Work out the finished part from the listing and answer in its coordinate system (mm). A direction names the side the tool comes from. Round coordinates to 2 decimals unless told otherwise and drop trailing zeros. Write each loop counter-clockwise with the first axis right and the second up, starting at its lowest first coordinate (ties: lowest second). Pieces come first, ordered by that corner, then holes. Notation, with made-up numbers: (19.25, -2.5) -> (34.25, -2.5) arc R7 cw to (34.25, 2.5) -> close; hole circle Ø1 at (55, -15.5). An arc over 180 degrees is marked (long way). One line per question, with ' | ' between items. Start each with the question number.
```python
from build123d import *

# Parameters (mm, degrees)
SKETCH2_R           = 23
CUT_EXTRUDE1_DEPTH  = 5
CUT_EXTRUDE2_START  = -2
SKETCH3_R           = 23
CUT_EXTRUDE2_DEPTH  = 2
SKETCH4_R           = 6
BOSS_EXTRUDE2_DEPTH = 5
CUT_EXTRUDE3_DEPTH  = 5
SKETCH6_R           = 1.5
CUT_EXTRUDE4_DEPTH  = 3
SKETCH7_RX          = 4
SKETCH7_RY          = 2.5
CUT_EXTRUDE5_DEPTH  = 3
CIRPATTERN1_COUNT   = 12


with BuildPart() as part:
    # Sketch1 → Revolve1 (revolve)
    with BuildSketch(Plane(origin=(0, 0, 0), x_dir=(1, 0, 0), z_dir=(0, 1, 0)), mode=Mode.PRIVATE) as revolve1_sk:
        Polygon((-5, 25), (0.5, 25), (0.5, 26.5), (0, 26.5), (0, 28), (3, 28), (3, 26.5), (2.5, 26.5), (2.5, 25), (5, 25), (5, 0), (-5, 0), align=None)
    revolve(revolve1_sk.sketch.rotate(Axis((0, 0, 0), (1, 0, 0)), 180), axis=Axis((0, 0, 0), (1, 0, 0)))

    # Sketch2 → Cut-Extrude1 (cut)
    with BuildSketch(Plane(origin=(5, 0, 0), x_dir=(0, 0, -1), z_dir=(1, 0, 0))):
        Circle(SKETCH2_R)
    extrude(amount=-CUT_EXTRUDE1_DEPTH, mode=Mode.SUBTRACT)

    # Sketch3 → Cut-Extrude2 (cut)
    with BuildSketch(Plane.ZY.offset(5).offset(CUT_EXTRUDE2_START)):
        with Locations(Location((0, 0, 0), (0, 0, 180))):
            Circle(SKETCH3_R)
    extrude(amount=CUT_EXTRUDE2_DEPTH, mode=Mode.SUBTRACT)

    # Sketch4 → Boss-Extrude2 (add)
    with BuildSketch(Plane(origin=(0, 0, 0), x_dir=(0, 0, -1), z_dir=(1, 0, 0))):
        with Locations(Location((0, 0, 0), (0, 0, 180))):
            Circle(SKETCH4_R)
    extrude(amount=BOSS_EXTRUDE2_DEPTH)

    # Sketch5 → Cut-Extrude3 (cut)
    with BuildSketch(Plane(origin=(5, 0, 0), x_dir=(0, 0, -1), z_dir=(1, 0, 0))):
        with BuildLine():
            Line((-1.936491673, 3.5), (1.936491673, 3.5))
            ThreePointArc((1.936491673, 3.5), (0, -4), (-1.936491673, 3.5))
        make_face()
    extrude(amount=-CUT_EXTRUDE3_DEPTH, mode=Mode.SUBTRACT)

    # Sketch6 → Cut-Extrude4 (cut)
    with BuildSketch(Plane.ZY.offset(3)):
        Circle(SKETCH6_R)
    extrude(amount=-CUT_EXTRUDE4_DEPTH, mode=Mode.SUBTRACT)

    # Sketch7 → Cut-Extrude5 (cut)
    with BuildSketch(Plane(origin=(0, 0, 0), x_dir=(0, 0, -1), z_dir=(1, 0, 0))):
        with Locations(Location((0, 15), (0, 0, -90))):
            Ellipse(SKETCH7_RX, SKETCH7_RY)
    cut_extrude5 = extrude(amount=-CUT_EXTRUDE5_DEPTH, mode=Mode.SUBTRACT)

    # CirPattern1: Cut-Extrude5 ×12 about axis
    cirpattern1_axis = Axis((4.242640687, 0, 0), (-1, 0, 0))
    for i in range(1, CIRPATTERN1_COUNT):
        add(cut_extrude5.rotate(cirpattern1_axis, i * 360 / CIRPATTERN1_COUNT), mode=Mode.SUBTRACT)


solid = part.part
```
(1) A cutting plane is placed at D-D, the plane y = 0. Count the separate pieces of the cut face and the enclosed holes in it, then the cut area to 3 significant figures.
(2) A cutting plane is placed at C-C, the plane z = -21.5. Determine the outline of the cut face in (x, y).
(3) Consider L1, parallel to Y at x = -1.8, z = 0; L2, parallel to Z at x = -1.5, y = 14.5; L3, parallel to Z at x = -1.5, y = -9. Determine where each line is inside the solid, lowest interval first.
(4) Given pin 1 Ø16 at (y, z) = (2.5, 9.5) entering from -X; pin 2 Ø4 at (x, z) = (1.5, 7.5) entering from +Y; pin 3 Ø12 at (y, z) = (4.5, 20.5) entering from -X; pin 4 Ø6 at (x, y) = (1.5, -21.5) entering from -Z, each flat-ended and moving along its own axis, determine where each tip first touches the part or whether it passes through.
(5) A cutting plane is placed at A-A, the plane x = 4. Determine the outline of the cut face in (y, z).
(6) A cutting plane is placed at B-B, the plane y = -22. Determine the outline of the cut face in (x, z).
(7) The mould has two halves that part along Z. Classify faces 1 (the flat face through (0, -5, -5)), 2 (the cylindrical face through (1.521, 10.724, 25.865)), 3 (the cylindrical face through (3.768, -7.509, 23.846)), 4 (the flat face through (5, 4, 0)): +Z half, -Z half, draft (parallel to the pull), parting line (faces both ways), or undercut.
(8) For faces 5 (the cylindrical face through (-3.986, -22.804, 2.994)), 6 (the cylindrical face through (2.535, 22.804, 2.994)), 7 (the flat face through (5, 22.1, 7.3)), determine the directions among +Z, -Z, +X, -X, +Y, -Y from which every point of the face is accessible in a straight line to the end or side of a thin tool.
Returned:
1) separate pieces: 4 | enclosed holes: 0 | area: 156 mm2
2) outline: (-5, -12.76) -> (0.5, -12.76) -> (0.5, -15.49) -> (0, -15.49) -> (0, -17.94) -> (3, -17.94) -> (3, -15.49) -> (2.5, -15.49) -> (2.5, -12.76) -> (5, -12.76) -> (5, -8.17) -> (0, -8.17) -> (0, 8.17) -> (5, 8.17) -> (5, 12.76) -> (2.5, 12.76) -> (2.5, 15.49) -> (3, 15.49) -> (3, 17.94) -> (0, 17.94) -> (0, 15.49) -> (0.5, 15.49) -> (0.5, 12.76) -> (-5, 12.76) -> (-5, 8.17) -> (-3, 8.17) -> (-3, -8.17) -> (-5, -8.17) -> close
3) L1: -25 to -19, -11 to -1.5, 1.5 to 11, 19 to 25 | L2: -20.37 to -10.45, -5.49 to -2.48, 2.48 to 5.49, 10.45 to 20.37 | L3: -23.32 to -16.64, -10.8 to 10.8, 16.64 to 23.32
4) pin 1: x = -3 | pin 2: y = 27.45 | pin 3: x = -5 | pin 4: z = -21.02
5) outline: circle Ø50 at (0, 0); circle Ø12 at (0, 0); hole circle Ø46 at (0, 0); hole (3.5, -1.94) -> (3.5, 1.94) arc R4 ccw (long way) to start
6) outline: (-5, -11.87) -> (0.5, -11.87) -> (0.5, -14.77) -> (0, -14.77) -> (0, -17.32) -> (3, -17.32) -> (3, -14.77) -> (2.5, -14.77) -> (2.5, -11.87) -> (5, -11.87) -> (5, -6.71) -> (0, -6.71) -> (0, 6.71) -> (5, 6.71) -> (5, 11.87) -> (2.5, 11.87) -> (2.5, 14.77) -> (3, 14.77) -> (3, 17.32) -> (0, 17.32) -> (0, 14.77) -> (0.5, 14.77) -> (0.5, 11.87) -> (-5, 11.87) -> (-5, 6.71) -> (-3, 6.71) -> (-3, -6.71) -> (-5, -6.71) -> close
7) face 1: undercut | face 2: parting line | face 3: undercut | face 4: draft
8) face 5: -X | face 6: +X | face 7: +Z, -Z, +X, +Y, -Y
